```python
from build123d import *
from OCP.BRepAlgoAPI import BRepAlgoAPI_Cut
from OCP.TopTools import TopTools_ListOfShape

# Parameters (mm, degrees)
BOSS_EXTRUDE6_DEPTH      = 2.5
CUT_EXTRUDE1_DEPTH       = 30.06261
CUT_EXTRUDE1_DEPTH_BACK  = 1.5
BOSS_EXTRUDE7_DEPTH      = 18.5
BOSS_EXTRUDE7_DEPTH_BACK = 1.5
CUT_EXTRUDE2_DEPTH       = 32.362831921
CUT_EXTRUDE2_DEPTH_BACK  = 32.362831921
SKETCH14_R               = 0.75
BOSS_EXTRUDE9_START      = 4.44
SKETCH19_W               = 1.5
SKETCH19_H               = 4
BOSS_EXTRUDE9_DEPTH      = 4.44
SKETCH21_W               = 1.5
SKETCH21_H               = 3
BOSS_EXTRUDE11_DEPTH     = 10
CUT_EXTRUDE3_DEPTH       = 34.819018318
CUT_EXTRUDE3_DEPTH_BACK  = 34.819018318
CUT_EXTRUDE4_DEPTH       = 32.833480802
CUT_EXTRUDE4_DEPTH_BACK  = 32.833480802


with BuildPart() as part:
    # Sketch9 → Boss-Extrude6 (new body)
    with BuildSketch(Plane(origin=(0, 3.23, 0), x_dir=(1, 0, 0), z_dir=(0, 1, 0))):
        with BuildLine():
            Line((3, 25.18), (14, 25.18))
            ThreePointArc((14, 25.18), (17.181980515, 23.861980515), (18.5, 20.68))
            Line((18.5, 20.68), (18.5, 3))
            Line((18.5, 3), (17, 3))
            Line((17, 3), (17, 21))
            ThreePointArc((17, 21), (16.121320344, 23.121320344), (14, 24))
            Line((14, 24), (3, 24))
            ThreePointArc((3, 24), (0.878679656, 23.121320344), (0, 21))
            Line((0, 21), (0, 3))
            Line((0, 3), (-1.5, 3))
            Line((-1.5, 3), (-1.5, 21))
            ThreePointArc((-1.5, 21), (-0.073983127, 23.977063175), (3, 25.18))
        make_face()
    extrude(amount=-BOSS_EXTRUDE6_DEPTH)

    # Sketch7 → Cut-Extrude1 (cut, two sides: drawn at the far end of the back side and taken through both)
    with BuildSketch(Plane(origin=(0, 0, -25.18), x_dir=(-1, 0, 0), z_dir=(0, 0, -1)).offset(-CUT_EXTRUDE1_DEPTH_BACK)):
        with BuildLine():
            Line((-12.97, 3.23), (-4.03, 3.23))
            Line((-4.03, 3.23), (-4.03, 2.95))
            ThreePointArc((-4.03, 2.95), (-4.410761184, 2.030761184), (-5.33, 1.65))
            Line((-5.33, 1.65), (-11.67, 1.65))
            ThreePointArc((-11.67, 1.65), (-12.589238816, 2.030761184), (-12.97, 2.95))
            Line((-12.97, 2.95), (-12.97, 3.23))
        make_face()
    extrude(amount=CUT_EXTRUDE1_DEPTH + CUT_EXTRUDE1_DEPTH_BACK, mode=Mode.SUBTRACT)

    # Sketch12 → Boss-Extrude7 (add, two sides: drawn at the far end of the back side and taken through both)
    with BuildSketch(Plane(origin=(0, 0, 0), x_dir=(0, 0, -1), z_dir=(1, 0, 0)).offset(-BOSS_EXTRUDE7_DEPTH_BACK)):
        Polygon((6.787278953, 1.65), (1.644409133, 1.65), (1.644409133, 0.15), (8.72, 0.15), (25.18, 0.15), (25.18, 1.65), align=None)
    extrude(amount=BOSS_EXTRUDE7_DEPTH + BOSS_EXTRUDE7_DEPTH_BACK)

    # Sketch14 → Cut-Extrude2 (cut, two sides: drawn at the far end of the back side and taken through both)
    # profile 1 of 5: a face of its own
    with BuildSketch(Plane(origin=(0, 2.86, 0), x_dir=(1, 0, 0), z_dir=(0, 1, 0)).offset(-CUT_EXTRUDE2_DEPTH_BACK)):
        Polygon((14.01139117, 26.68), (3.013153393, 26.68), (2.986846607, 26.68), (-3, 26.68), (-3, 21.049560468), (-3, 3), (-3, -2.88), (-3, -8.88), (3, -8.88), (13.998237777, -8.88), (14.024544563, -8.88), (20, -8.88), (20, -3.249560468), (20, 2.630439532), (20, 20.68), (20, 26.68), align=None)
        with BuildLine():
            Line((14, -7.38), (3, -7.38))
            ThreePointArc((3, -7.38), (-0.181980515, -6.061980515), (-1.5, -2.88))
            Line((-1.5, -2.88), (-1.5, 3))
            Line((-1.5, 3), (-1.499971165, 20.691405551))
            ThreePointArc((-1.499971165, 20.691405551), (-0.177940395, 23.866009567), (3, 25.18))
            Line((3, 25.18), (14, 25.18))
            ThreePointArc((14, 25.18), (17.181980515, 23.861980515), (18.5, 20.68))
            Line((18.5, 20.68), (18.5, 3))
            Line((18.5, 3), (18.5, -2.88))
            ThreePointArc((18.5, -2.88), (17.181980515, -6.061980515), (14, -7.38))
        make_face(mode=Mode.SUBTRACT)
    # profile 2 of 5: a face of its own
    with BuildSketch(Plane(origin=(0, 2.86, 0), x_dir=(1, 0, 0), z_dir=(0, 1, 0)).offset(-CUT_EXTRUDE2_DEPTH_BACK)):
        with Locations((4.75, 1.52)):
            Circle(SKETCH14_R)
    # profile 3 of 5: a face of its own
    with BuildSketch(Plane(origin=(0, 2.86, 0), x_dir=(1, 0, 0), z_dir=(0, 1, 0)).offset(-CUT_EXTRUDE2_DEPTH_BACK)):
        with Locations((7.25, 1.52)):
            Circle(SKETCH14_R)
    # profile 4 of 5: a face of its own
    with BuildSketch(Plane(origin=(0, 2.86, 0), x_dir=(1, 0, 0), z_dir=(0, 1, 0)).offset(-CUT_EXTRUDE2_DEPTH_BACK)):
        with Locations((9.75, 1.52)):
            Circle(SKETCH14_R)
    # profile 5 of 5: a face of its own
    with BuildSketch(Plane(origin=(0, 2.86, 0), x_dir=(1, 0, 0), z_dir=(0, 1, 0)).offset(-CUT_EXTRUDE2_DEPTH_BACK)):
        with Locations((12.25, 1.52)):
            Circle(SKETCH14_R)
    extrude(amount=CUT_EXTRUDE2_DEPTH + CUT_EXTRUDE2_DEPTH_BACK, mode=Mode.SUBTRACT)

    # Sketch19 → Boss-Extrude9 (add)
    with BuildSketch(Plane(origin=(0, 1.65, 0), x_dir=(1, 0, 0), z_dir=(0, 1, 0)).offset(BOSS_EXTRUDE9_START)):
        with BuildLine():
            Line((17, 21), (17, 16))
            Line((17, 16), (17, 7))
            Line((17, 7), (17, 3))
            Line((17, 3), (15.5, 3))
            Line((15.5, 3), (15.5, 7))
            Line((15.5, 7), (15.5, 16))
            Line((15.5, 16), (15.5, 21))
            ThreePointArc((15.5, 21), (15.060660172, 22.060660172), (14, 22.5))
            Line((14, 22.5), (14, 24))
            ThreePointArc((14, 24), (16.121320344, 23.121320344), (17, 21))
        make_face()
        with BuildLine():
            Line((0, 21), (0, 16))
            Line((0, 16), (1.5, 16))
            Line((1.5, 16), (1.5, 21))
            ThreePointArc((1.5, 21), (1.939339828, 22.060660172), (3, 22.5))
            Line((3, 22.5), (3, 24))
            ThreePointArc((3, 24), (0.878679656, 23.121320344), (0, 21))
        make_face()
        with Locations((0.75, 5)):
            Rectangle(SKETCH19_W, SKETCH19_H)
    extrude(amount=-BOSS_EXTRUDE9_DEPTH)

    # Sketch21 → Boss-Extrude11 (add)
    with BuildSketch(Plane.XY.offset(-16)):
        with Locations((0.75, 3.15)):
            Rectangle(SKETCH21_W, SKETCH21_H)
    extrude(amount=BOSS_EXTRUDE11_DEPTH)


with BuildPart() as cut_extrude3_tool:
    # Sketch17 → Cut-Extrude3 (new, two sides: drawn at the far end of the back side and taken through both)
    with BuildSketch(Plane(origin=(0, -6.85, 0), x_dir=(-1, 0, 0), z_dir=(0, -1, 0)).offset(-CUT_EXTRUDE3_DEPTH_BACK)):
        with BuildLine():
            Line((-14.620622145, 8.72), (-2.379377855, 8.72))
            ThreePointArc((-2.379377855, 8.72), (0.394318757, 7.217422785), (1.5, 4.263002339))
            Line((1.5, 4.263002339), (1.5, -1.5))
            Line((1.5, -1.5), (-18.5, -1.5))
            Line((-18.5, -1.5), (-18.5, 4.263002339))
            ThreePointArc((-18.5, 4.263002339), (-17.394318757, 7.217422785), (-14.620622145, 8.72))
        make_face()
    extrude(amount=CUT_EXTRUDE3_DEPTH + CUT_EXTRUDE3_DEPTH_BACK)


with BuildPart() as part_1:
    add(part.part)

    # Cut-Extrude3: cut by cut_extrude3_tool, with a tolerance
    cut_extrude3_stock = TopTools_ListOfShape()
    cut_extrude3_stock.Append(part_1.part.wrapped)
    cut_extrude3_tools = TopTools_ListOfShape()
    cut_extrude3_tools.Append(cut_extrude3_tool.part.wrapped)
    cut_extrude3_cut = BRepAlgoAPI_Cut()
    cut_extrude3_cut.SetArguments(cut_extrude3_stock)
    cut_extrude3_cut.SetTools(cut_extrude3_tools)
    cut_extrude3_cut.SetFuzzyValue(0.00001)
    cut_extrude3_cut.Build()
    add(Compound.cast(cut_extrude3_cut.Shape()).solids(), mode=Mode.REPLACE)

    # Sketch20 → Cut-Extrude4 (cut, two sides: drawn at the far end of the back side and taken through both)
    with BuildSketch(Plane(origin=(0, 0, 0), x_dir=(0, 0, -1), z_dir=(1, 0, 0)).offset(-CUT_EXTRUDE4_DEPTH_BACK)):
        with BuildLine():
            Line((-1.38, 1.65), (0.12, 1.65))
            Line((0.12, 1.65), (2.72, 1.65))
            ThreePointArc((2.72, 1.65), (4.841320344, 0.771320344), (5.72, -1.35))
            Line((5.72, -1.35), (5.72, -6.35))
            Line((5.72, -6.35), (5.72, -7.888681431))
            Line((5.72, -7.888681431), (-4.38, -7.888681431))
            Line((-4.38, -7.888681431), (-4.38, -6.35))
            Line((-4.38, -6.35), (-4.38, -1.35))
            ThreePointArc((-4.38, -1.35), (-3.501320344, 0.771320344), (-1.38, 1.65))
        make_face()
    extrude(amount=CUT_EXTRUDE4_DEPTH + CUT_EXTRUDE4_DEPTH_BACK, mode=Mode.SUBTRACT)


solid = part_1.part
```
Can you work these out from the model? Positions are in its coordinate system, mm. A direction names the side the tool comes from. Coordinates: 2 decimals unless noted, no trailing zeros. Loops run counter-clockwise (first coordinate to the right, second up) from the corner with the lowest first, then second, coordinate; pieces in that order, holes last. Notation, with made-up numbers: (18.5, -9.75) - (22.5, -9.75) arc R6 ccw to (22.5, -2.75) - close; hole circle Ø10 at (62, 84). An arc over 180 degrees is marked (long way). Answer as CSV lines item,"result". Start each with the question number.
1) Suppose I cut it at B-B (z = -19). Please give me the cut outline in (x, y).
2) I need wall thicknesses on line 1 (X direction, y = 2.65, z = -13); line 2 (Y direction, x = 7.25, z = -20); line 3 (Y direction, x = 1, z = -11.75). Which ranges of each line are inside material? Lowest first, please. Write a range as from..to.
3) For pin 1 (1.5 mm diameter, centred on x = 14, y = 5.5, fed in from -Z); pin 2 (2 mm diameter, centred on x = 0.5, y = 3, fed in from -Z); pin 3 (1.3 mm diameter, centred on x = 13, y = 2, fed in from +Z), each with a flat end and sliding along its axis, tell me the tip position at first contact or that it passes through.
4) Suppose I cut it at D-D (x = 1). Please give me the cut outline in (y, z), plus the area to 3 significant figures.
5) Thinking about a two-plate mould opening in X: for faces 5 (the flat face through (3, 4, -23)), 6 (the cylindrical face through (17.147, 1.668, -23.897)), 7 (the flat face through (9, 1, -8.72)), 8 (the flat face through (17.2, 3.23, -17.1)), which applies, pulls with the +X half, pulls with the -X half, needs draft (parallel to the pull), parting line crosses it, or undercut?
6) Which directions (+Z, -Z, +X, -X, +Y, -Y) give clear straight access to the entire face, cutting with the end or side of a thin tool? Please do faces 1 (the cylindrical face through (0.9, 4.68, -23.14)), 2 (the cylindrical face through (17.424, 2.502, -7.183)), 3 (the flat face through (1, 5, -16)), 4 (the cylindrical face through (1.93, 3.9, -22.05)).
7) Suppose I cut it at C-C (y = 5.35). Please give me the cut outline in (x, z), plus the area to 3 significant figures.
8) Suppose I cut it at A-A (y = 4.2). Please give me the cut outline in (x, z).
Check result:
1,outline,"(-1.5, 0.15) - (18.5, 0.15) - (18.5, 3.23) - (17, 3.23) - (17, 6.09) - (15.5, 6.09) - (15.5, 1.65) - (1.5, 1.65) - (1.5, 6.09) - (0, 6.09) - (0, 3.23) - (-1.5, 3.23) - close"
2,line 1,"x = -1.5..1.5, 15.5..18.5"
2,line 2,"y = 0.15..1.65"
2,line 3,"y = 0.15..4.65"
3,pin 1,"stops at z = -24"
3,pin 2,"stops at z = -24.92"
3,pin 3,"stops at z = -8.72"
4,outline,"(0.15, -24.71) - (3.23, -24.71) - (3.23, -23.24) - (6.09, -23.24) - (6.09, -16) - (4.65, -16) - (4.65, -8.29) - (0.15, -8.29) - close"
4,area,"82.2 mm²"
5,face 5,"undercut"
5,face 6,"pulls with the +X half"
5,face 7,"undercut"
5,face 8,"needs draft"
6,face 1,"-Z, -X, +Y"
6,face 2,"+Z, +Y, -Y"
6,face 3,"+Z, -X, +Y"
6,face 4,"+Z, +Y"
7,outline,"(0, -21) arc R3 ccw to (3, -24) - (3, -22.5) arc R1.5 cw to (1.5, -21) - (1.5, -16) - (0, -16) - close; (14, -24) arc R3 ccw to (17, -21) - (17, -7.62) arc R4.5 cw to (15.5, -8.51) - (15.5, -21) arc R1.5 cw to (14, -22.5) - close"
7,area,"37.4 mm²"
8,outline,"(0, -21) arc R3 ccw to (3, -24) - (3, -22.5) arc R1.5 cw to (1.5, -21) - (1.5, -8.51) arc R4.5 cw to (0, -7.62) - close; (14, -24) arc R3 ccw to (17, -21) - (17, -7.62) arc R4.5 cw to (15.5, -8.51) - (15.5, -21) arc R1.5 cw to (14, -22.5) - close"
